```python
from build123d import *

# Parameters (mm, degrees)
F1_DEPTH  = 7
F2_W      = 32
F2_H      = 3
F3_DEPTH  = 25
F4_R      = 8.5
F5_DEPTH  = 3.3
F6_R      = 6.25
F7_DEPTH  = 5.7
F8_R      = 8.25
F9_DEPTH  = 4
F10_R     = 6
F11_DEPTH = 50
F12_DEPTH = 5


with BuildPart() as f1:
    # F0 (on Front) → F1 (new body)
    with BuildSketch(Plane.XZ):
        Polygon((-16, 0), (0, 0), (16, 0), (16, 6), (22, 6), (22, 71), (0, 71), (-22, 71), (-22, 6), (-16, 6), align=None)
    extrude(amount=F1_DEPTH)

    # F2 (on face) → F3 (join)
    with BuildSketch(Plane(origin=(0, 0, 0), x_dir=(1, 0, 0), z_dir=(0, 0, -1))):
        with Locations((0, 8.5)):
            Rectangle(F2_W, F2_H)
    extrude(amount=-F3_DEPTH)

    # F4 (on face) → F5 (cut)
    with BuildSketch(Plane(origin=(0, 0, 0), x_dir=(1, 0, 0), z_dir=(0, 0, -1))):
        with Locations((0, 10)):
            Circle(F4_R)
    extrude(amount=-F5_DEPTH, mode=Mode.SUBTRACT)

    # F6 (on face) → F7 (cut)
    with BuildSketch(Plane(origin=(0, 0, 3.3), x_dir=(1, 0, 0), z_dir=(0, 0, -1))):
        with Locations((0, 10)):
            Circle(F6_R)
    extrude(amount=-F7_DEPTH, mode=Mode.SUBTRACT)

    # F8 (on face) → F9 (cut)
    with BuildSketch(Plane(origin=(0, 0, 9), x_dir=(1, 0, 0), z_dir=(0, 0, -1))):
        with Locations((0, 10)):
            Circle(F8_R)
    extrude(amount=-F9_DEPTH, mode=Mode.SUBTRACT)

    # F10 (on face) → F11 (cut)
    with BuildSketch(Plane(origin=(0, 0, 13), x_dir=(1, 0, 0), z_dir=(0, 0, -1))):
        with Locations((0, 10)):
            Circle(F10_R)
    extrude(amount=-F11_DEPTH, mode=Mode.SUBTRACT)

    # F12 (add): faces of the model
    f12_faces = [f1.faces().sort_by_distance(p)[0] for p in [
        (-11.3145331244, -10, 12.9844320761),
        (11.3145331244, -10, 12.9844320761),
    ]]
    extrude(f12_faces, amount=F12_DEPTH)


solid = f1.part
```
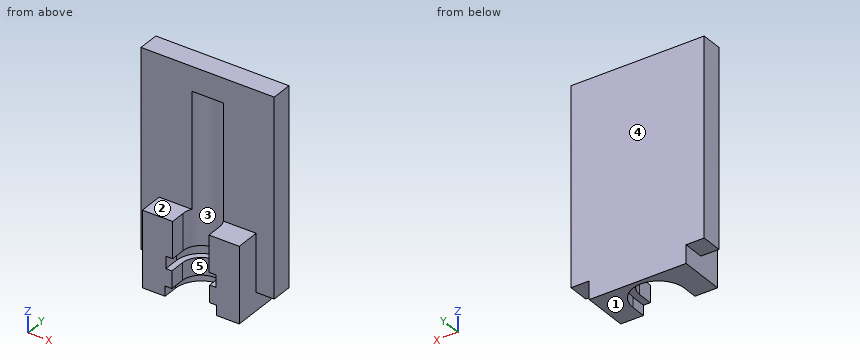
Input: part model. Units: mm. Frame: model coordinates. Face numbers are marked on the shaded views. A direction names the side the tool comes from. Give positions to 0.01 mm unless a question says otherwise; leave off trailing zeros. Write each loop counter-clockwise with the first axis right and the second up, starting at its lowest first coordinate (ties: lowest second). Pieces come first, ordered by that corner, then holes. Notation, with made-up numbers: (11.25, 86) - (33.25, 86) arc R21 cw to (33.25, 121) - close; hole circle Ø9 at (-8.75, 30). An arc over 180 degrees is marked (long way). Write item = value, one per line. Start each with the question number.
1. Section query B-B, the plane z = 22. Output: boundary loops of the cut face in (x, y), then the cut area to 3 significant figures.
2. Ray query, L1, parallel to X at y = -13, z = 7; L2, parallel to X at y = -13.75, z = 24; L3, parallel to Y at x = -18.5, z = 28.5. Return the intervals inside material, ascending.
3. Section query A-A, the plane y = -12.5. Output: boundary loops of the cut face in (x, z).
4. Section query C-C, the plane x = 0. Output: boundary loops of the cut face in (y, z), then the cut area to 3 significant figures.
5. Section query D-D, the plane y = -2.75. Output: boundary loops of the cut face in (x, z).
6. Access query for the marked faces 1 and 2. Directions: +Z, -Z, +X, -X, +Y, -Y. A direction counts if a zero-diameter tool reaches every point of the face in a straight line with its end or side. Return the directions, or none.
7. First-contact query: pin 1 Ø3.5 at (x, y) = (-2, -5) entering from -Z; pin 2 Ø3 at (x, y) = (-18.5, -4.5) entering from -Z; pin 3 Ø4 at (y, z) = (-13.5, 5) entering from +X. Flat tips, straight axial feed; report the tip coordinate or a pass-through.
8. Mould query, pull axis X, two halves, no side actions, for the marked faces 3, 4 and 5. Classes: released by +X, released by -X, zero draft, split by the parting line, or undercut.
Check sheet entries:
q1.outline = (-22, -7) - (-16, -7) - (-16, -15) - (-6, -15) - (-6, -10) arc R6 cw to (6, -10) - (6, -15) - (16, -15) - (16, -7) - (22, -7) - (22, 0) - (-22, 0) - close
q1.area = 447 mm2
q2.L1 = -16 to -6.25, 6.25 to 16
q2.L2 = -16 to -6, 6 to 16
q2.L3 = -7 to 0
q3.outline = (-16, 0) - (-8.5, 0) - (-8.5, 3.3) - (-6.25, 3.3) - (-6.25, 9) - (-8.25, 9) - (-8.25, 13) - (-6, 13) - (-6, 25) - (-16, 25) - close; (6, 13) - (8.25, 13) - (8.25, 9) - (6.25, 9) - (6.25, 3.3) - (8.5, 3.3) - (8.5, 0) - (16, 0) - (16, 25) - (6, 25) - close
q4.outline = (-7, 63) - (-4, 63) - (-4, 13) - (-1.75, 13) - (-1.75, 9) - (-3.75, 9) - (-3.75, 3.3) - (-1.5, 3.3) - (-1.5, 0) - (0, 0) - (0, 71) - (-7, 71) - close
q4.area = 289 mm2
q5.outline = (-22, 6) - (-16, 6) - (-16, 0) - (-4.44, 0) - (-4.44, 3.3) - (4.44, 3.3) - (4.44, 0) - (16, 0) - (16, 6) - (22, 6) - (22, 71) - (-22, 71) - close; hole (-3.94, 9) - (3.94, 9) - (3.94, 13) - (-3.94, 13) - close
q6.face_1 = -Z, +X, -X, +Y, -Y
q6.face_2 = +Z, +X, -X, -Y
q7.pin_1 = 3.3
q7.pin_2 = 6
q7.pin_3 = 16
q8.face_3 = undercut
q8.face_4 = zero draft
q8.face_5 = undercut
